Source: CAD feature listing. Evaluate the final solid. Frame: model axes, mm. Face numbers are marked on the shaded views. A direction names the side the tool comes from. Round coordinates to 2 decimals unless told otherwise and drop trailing zeros. Loops run counter-clockwise (first coordinate to the right, second up) from the corner with the lowest first, then second, coordinate; pieces in that order, holes last. Notation, with made-up numbers: (37.25, 29) -> (81.25, 29) arc R29 ccw to (81.25, 63) -> close; hole circle Ø1 at (-8.75, -8.75). An arc over 180 degrees is marked (long way). Write item = value, one per line.
from build123d import *
from OCP.BRepFilletAPI import BRepFilletAPI_MakeChamfer

# Parameters (mm, degrees)
SKETCH1_R                  = 2.2
SKETCH1_W                  = 22.4
SKETCH1_H                  = 25.8
BOSS_EXTRUDE1_DEPTH        = 42
CUT_EXTRUDE1_DEPTH         = 69.433909723
BOSS_EXTRUDE2_DEPTH        = 14.6
SKETCH4_W                  = 36
SKETCH4_H                  = 20
CUT_EXTRUDE2_DEPTH         = 18.2
SKETCH5_R                  = 2.2
CUT_EXTRUDE3_DEPTH         = 71.161242862
SKETCH16_W                 = 26.03
SKETCH16_H                 = 42
BOSS_EXTRUDE6_DEPTH        = 3
CHAMFER1_SIZE              = 7.42526056
CHAMFER1_SIZE_2            = 3
CHAMFER1_OF_MIRROR7_SIZE   = 7.42526056
CHAMFER1_OF_MIRROR7_SIZE_2 = 3
CUT_EXTRUDE4_START         = -1.9
CUT_EXTRUDE4_DEPTH         = 3.35
SKETCH10_R                 = 1.2
CUT_EXTRUDE10_DEPTH        = 72.637978754
SKETCH13_W                 = 22.4
SKETCH13_H                 = 1.9
BOSS_EXTRUDE4_DEPTH        = 1
SKETCH14_W                 = 3
SKETCH14_H                 = 7
CUT_EXTRUDE11_DEPTH        = 2.8
SKETCH15_W                 = 22.4
SKETCH15_H                 = 1.9
BOSS_EXTRUDE5_DEPTH        = 1
MIRROR5_START              = -1.9
MIRROR5_COPY_1_DEPTH       = 3.35
SKETCH17_W                 = 13.216816462
SKETCH17_H                 = 5
SKETCH17_W_2               = 8
BOSS_EXTRUDE7_DEPTH        = 3.2
FILLET1_SIZE               = 3
FILLET1_SIZE_2             = 18
FILLET3_SIZE               = 5
FILLET3_SIZE_2             = 4


# Some blends are built 0.0001 mm under size
with BuildPart() as part:
    # Sketch1 → Boss-Extrude1 (new body)
    with BuildSketch(Plane.XY):
        Polygon((2, 0), (45.2, 0), (45.2, 29.6), (2, 29.6), (0, 29.6), (0, 27.6), (0, 2), (0, 0), align=None)
        with Locations(Location((35.2, 14.8, 0), (0, 0, 180))):
            Circle(SKETCH1_R, mode=Mode.SUBTRACT)
        with Locations((13, 14.8)):
            Rectangle(SKETCH1_W, SKETCH1_H, mode=Mode.SUBTRACT)
    extrude(amount=BOSS_EXTRUDE1_DEPTH)

    # Sketch2 → Cut-Extrude1 (cut, through all)
    with BuildSketch(Plane(origin=(0, 29.6, 0), x_dir=(1, 0, 0), z_dir=(0, 1, 0))):
        Polygon((45.2, -26), (26.03, -42), (45.2, -42), align=None)
    extrude(amount=-CUT_EXTRUDE1_DEPTH, mode=Mode.SUBTRACT)

    # Sketch3 → Boss-Extrude2 (add)
    with BuildSketch(Plane(origin=(0, 0, 0), x_dir=(-1, 0, 0), z_dir=(0, 0, -1))):
        Polygon((-38.8, 0), (-45.2, -3.8), (-45.2, 0), align=None)
        Polygon((-45.2, 29.6), (-38.8, 29.6), (-45.2, 33.4), align=None)
    extrude(amount=-BOSS_EXTRUDE2_DEPTH)

    # Sketch4 → Cut-Extrude2 (cut)
    with BuildSketch(Plane(origin=(45.2, 0, 0), x_dir=(0, 0, -1), z_dir=(1, 0, 0))):
        with Locations((-24, 14.8)):
            Rectangle(SKETCH4_W, SKETCH4_H)
    extrude(amount=-CUT_EXTRUDE2_DEPTH, mode=Mode.SUBTRACT)

    # Sketch5 → Cut-Extrude3 (cut, through all)
    with BuildSketch(Plane(origin=(0, 29.6, 0), x_dir=(1, 0, 0), z_dir=(0, 1, 0))):
        with Locations(Location((35.2, -16, 0), (0, 0, 270))):
            Circle(SKETCH5_R)
    extrude(amount=-CUT_EXTRUDE3_DEPTH, mode=Mode.SUBTRACT)

    # Sketch16 → Boss-Extrude6 (add)
    with BuildSketch(Plane(origin=(0, 29.6, 0), x_dir=(1, 0, 0), z_dir=(0, 1, 0))):
        with Locations((13.015, -21)):
            Rectangle(SKETCH16_W, SKETCH16_H)
    boss_extrude6 = extrude(amount=BOSS_EXTRUDE6_DEPTH)

    # Chamfer1
    chamfer1_edges_1 = [part.edges().sort_by_distance(p)[0] for p in [
        (13.015, 32.6, 42),
    ]]
    chamfer1_side_1 = [part.faces().sort_by_distance(p)[0] for p in [
        (13.015, 32.6, 41.94),
    ]]
    chamfer1_edges_2 = [part.edges().sort_by_distance(p)[0] for p in [
        (26.03, 32.6, 21),
    ]]
    chamfer1_side_2 = [part.faces().sort_by_distance(p)[0] for p in [
        (26.03, 32.54, 21),
    ]]
    chamfer1_edges_3 = [part.edges().sort_by_distance(p)[0] for p in [
        (13.015, 32.6, 0),
    ]]
    chamfer1_side_3 = [part.faces().sort_by_distance(p)[0] for p in [
        (13.015, 32.6, 0.06),
    ]]
    chamfer1_edges_4 = [part.edges().sort_by_distance(p)[0] for p in [
        (0, 32.6, 21),
    ]]
    chamfer1_side_4 = [part.faces().sort_by_distance(p)[0] for p in [
        (0.06, 32.6, 21),
    ]]
    chamfer1 = BRepFilletAPI_MakeChamfer(part.part.solid().wrapped)
    for e in chamfer1_edges_1:
        chamfer1.Add(CHAMFER1_SIZE - 0.0001, CHAMFER1_SIZE_2 - 0.0001, e.wrapped, chamfer1_side_1[0].wrapped)
    for e in chamfer1_edges_2:
        chamfer1.Add(CHAMFER1_SIZE_2 - 0.0001, CHAMFER1_SIZE - 0.0001, e.wrapped, chamfer1_side_2[0].wrapped)
    for e in chamfer1_edges_3:
        chamfer1.Add(CHAMFER1_SIZE - 0.0001, CHAMFER1_SIZE_2 - 0.0001, e.wrapped, chamfer1_side_3[0].wrapped)
    for e in chamfer1_edges_4:
        chamfer1.Add(CHAMFER1_SIZE - 0.0001, CHAMFER1_SIZE_2 - 0.0001, e.wrapped, chamfer1_side_4[0].wrapped)
    add(Compound.cast(chamfer1.Shape()), mode=Mode.REPLACE)  # a hair under: the kernel refuses the full size

    # Mirror7: Boss-Extrude6 across plane
    add(boss_extrude6.mirror(Plane(origin=(0, 14.8, 0), x_dir=(0, 0, 1), z_dir=(0, -1, 0))))

    # Chamfer1 of Mirror7
    chamfer1_of_mirror7_edges_1 = [part.edges().sort_by_distance(p)[0] for p in [
        (13.015, -3, 42),
    ]]
    chamfer1_of_mirror7_side_1 = [part.faces().sort_by_distance(p)[0] for p in [
        (13.015, -3, 41.94),
    ]]
    chamfer1_of_mirror7_edges_2 = [part.edges().sort_by_distance(p)[0] for p in [
        (26.03, -3, 21),
    ]]
    chamfer1_of_mirror7_side_2 = [part.faces().sort_by_distance(p)[0] for p in [
        (26.03, -2.94, 21),
    ]]
    chamfer1_of_mirror7_edges_3 = [part.edges().sort_by_distance(p)[0] for p in [
        (13.015, -3, 0),
    ]]
    chamfer1_of_mirror7_side_3 = [part.faces().sort_by_distance(p)[0] for p in [
        (13.015, -2.94, 0),
    ]]
    chamfer1_of_mirror7_edges_4 = [part.edges().sort_by_distance(p)[0] for p in [
        (0, -3, 21),
    ]]
    chamfer1_of_mirror7_side_4 = [part.faces().sort_by_distance(p)[0] for p in [
        (0.06, -3, 21),
    ]]
    chamfer1_of_mirror7 = BRepFilletAPI_MakeChamfer(part.part.solid().wrapped)
    for e in chamfer1_of_mirror7_edges_1:
        chamfer1_of_mirror7.Add(CHAMFER1_OF_MIRROR7_SIZE - 0.0001, CHAMFER1_OF_MIRROR7_SIZE_2 - 0.0001, e.wrapped, chamfer1_of_mirror7_side_1[0].wrapped)
    for e in chamfer1_of_mirror7_edges_2:
        chamfer1_of_mirror7.Add(CHAMFER1_OF_MIRROR7_SIZE_2 - 0.0001, CHAMFER1_OF_MIRROR7_SIZE - 0.0001, e.wrapped, chamfer1_of_mirror7_side_2[0].wrapped)
    for e in chamfer1_of_mirror7_edges_3:
        chamfer1_of_mirror7.Add(CHAMFER1_OF_MIRROR7_SIZE_2 - 0.0001, CHAMFER1_OF_MIRROR7_SIZE - 0.0001, e.wrapped, chamfer1_of_mirror7_side_3[0].wrapped)
    for e in chamfer1_of_mirror7_edges_4:
        chamfer1_of_mirror7.Add(CHAMFER1_OF_MIRROR7_SIZE - 0.0001, CHAMFER1_OF_MIRROR7_SIZE_2 - 0.0001, e.wrapped, chamfer1_of_mirror7_side_4[0].wrapped)
    add(Compound.cast(chamfer1_of_mirror7.Shape()), mode=Mode.REPLACE)  # a hair under: the kernel refuses the full size

    # Sketch6 → Cut-Extrude4 (cut)
    with BuildSketch(Plane(origin=(0, 29.6, 0), x_dir=(1, 0, 0), z_dir=(0, 1, 0)).offset(CUT_EXTRUDE4_START)):
        Polygon((11.35, -13.4), (9.775198425, -10.5), (11.35, -7.6), (14.65, -7.6), (16.244163906, -10.5), (14.65, -13.4), align=None)
    cut_extrude4 = extrude(amount=CUT_EXTRUDE4_DEPTH, mode=Mode.SUBTRACT)

    # Sketch10 → Cut-Extrude10 (cut, through all)
    with BuildSketch(Plane(origin=(0, 32.6, 0), x_dir=(1, 0, 0), z_dir=(0, 1, 0))):
        with Locations(Location((13, -10.4, 0), (0, 0, 270))):
            Circle(SKETCH10_R)
    cut_extrude10 = extrude(amount=-CUT_EXTRUDE10_DEPTH, mode=Mode.SUBTRACT)

    # Mirror4: Cut-Extrude4 across plane
    add(cut_extrude4.mirror(Plane(origin=(0, 14.8, 0), x_dir=(0, 0, 1), z_dir=(0, -1, 0))), mode=Mode.SUBTRACT)

    # Sketch13 → Boss-Extrude4 (add)
    with BuildSketch(Plane.XY.offset(42)):
        with Locations((13, 2.85)):
            Rectangle(SKETCH13_W, SKETCH13_H)
        with Locations((13, 26.75)):
            Rectangle(SKETCH13_W, SKETCH13_H)
    extrude(amount=-BOSS_EXTRUDE4_DEPTH)

    # Sketch14 → Cut-Extrude11 (cut)
    with BuildSketch(Plane(origin=(27, 0, 0), x_dir=(0, 0, -1), z_dir=(1, 0, 0))):
        with Locations((-9.5, 14.8)):
            Rectangle(SKETCH14_W, SKETCH14_H)
        with Locations((-22.5, 14.8)):
            Rectangle(SKETCH14_W, SKETCH14_H)
    extrude(amount=-CUT_EXTRUDE11_DEPTH, mode=Mode.SUBTRACT)

    # Sketch15 → Boss-Extrude5 (add)
    with BuildSketch(Plane(origin=(0, 0, 0), x_dir=(-1, 0, 0), z_dir=(0, 0, -1))):
        with Locations((-13, 2.85)):
            Rectangle(SKETCH15_W, SKETCH15_H)
        with Locations((-13, 26.75)):
            Rectangle(SKETCH15_W, SKETCH15_H)
    extrude(amount=-BOSS_EXTRUDE5_DEPTH)

    # Mirror5: Cut-Extrude4, Cut-Extrude10 across plane
    add(cut_extrude4.mirror(Plane.XY.offset(21)), mode=Mode.SUBTRACT)
    add(cut_extrude10.mirror(Plane.XY.offset(21)), mode=Mode.SUBTRACT)

    # Mirror5 copy 1 sketch → Mirror5 copy 1 (cut)
    with BuildSketch(Plane(origin=(0, 0, 42), x_dir=(1, 0, 0), z_dir=(0, -1, 0)).offset(MIRROR5_START)):
        Polygon((11.35, -13.4), (9.775198425, -10.5), (11.35, -7.6), (14.65, -7.6), (16.244163906, -10.5), (14.65, -13.4), align=None)
    extrude(amount=MIRROR5_COPY_1_DEPTH, mode=Mode.SUBTRACT)

    # Sketch17 → Boss-Extrude7 (add)
    with BuildSketch(Plane.ZY.offset(-24.2)):
        with Locations((30.608408231, 14.8)):
            Rectangle(SKETCH17_W, SKETCH17_H)
        with Locations((4, 14.8)):
            Rectangle(SKETCH17_W_2, SKETCH17_H)
    extrude(amount=BOSS_EXTRUDE7_DEPTH)

    # Fillet1
    # a fillet whose section is not a circle: 18, 3 mm, written as the material it takes off along each edge
    with BuildSketch(Plane(origin=(21, 12.3, 24), x_dir=(1, 0, 0), z_dir=(0, 1, 0))) as fillet1_piece_1:
        with BuildLine():
            Bezier((FILLET1_SIZE, 0), (0, 0), (0, -FILLET1_SIZE_2), weights=[1, 0.538461538, 1])
            Line((0, -FILLET1_SIZE_2), (0, 0))
            Line((0, 0), (FILLET1_SIZE, 0))
        make_face()
    extrude(amount=5, mode=Mode.SUBTRACT)

    # Fillet2
    # a fillet whose section is not a circle: 1 mm, written as the material it takes off along each edge
    with BuildSketch(Plane(origin=(21.159285498, 19.997028117, 37.216816462), x_dir=(1, 0, 0), z_dir=(0, -1, 0))) as fillet2_piece_1:
        with BuildLine():
            Bezier((1.072400011, 0), (-0.006916058, 0), (0.075305906, -1.076179691), weights=[1, 1, 1])
            ThreePointArc((0.075305906, -1.076179691), (0.035933118, -0.538210194), (0, 0))
            Line((0, 0), (1.072400011, 0))
        make_face()
    extrude(amount=10.394056235, mode=Mode.SUBTRACT)

    # Fillet3
    # a fillet whose section is not a circle: 5, 4 mm, written as the material it takes off along each edge
    with BuildSketch(Plane(origin=(21, -0.2, 8), x_dir=(0, 0, -1), z_dir=(0, 1, 0))) as fillet3_piece_1_section:
        with BuildLine():
            Bezier((FILLET3_SIZE, 0), (0, 0), (0, -FILLET3_SIZE_2), weights=[1, 0.538461538, 1])
            Line((0, -FILLET3_SIZE_2), (0, 0))
            Line((0, 0), (FILLET3_SIZE, 0))
        make_face()
    fillet3_piece_1 = extrude(amount=30, mode=Mode.PRIVATE)
    fillet3_piece_1 = split(fillet3_piece_1, bisect_by=Plane(origin=(21, 18.3, 8), z_dir=(0, -1, 0)), keep=Keep.TOP, mode=Mode.PRIVATE)
    fillet3_piece_1 = split(fillet3_piece_1, bisect_by=Plane(origin=(21, 11.3, 8), z_dir=(0, 1, 0)), keep=Keep.TOP, mode=Mode.PRIVATE)
    add(fillet3_piece_1, mode=Mode.SUBTRACT)


solid = part.part
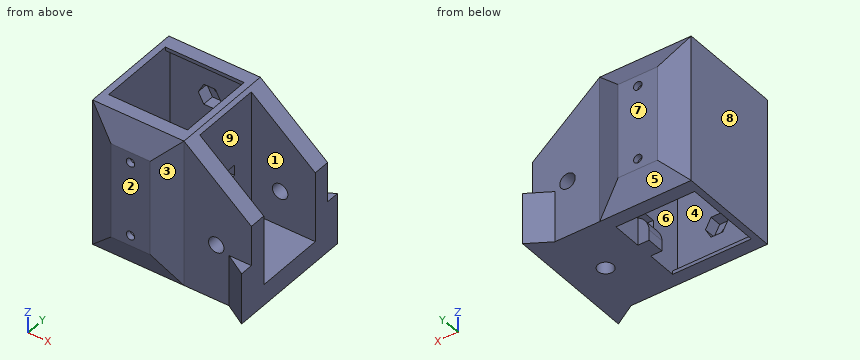
1. Section query A-A (z = 16). Give the number of separate pieces and of enclosed holes in the cut face, then the cut area to 3 significant figures.
Evaluation:
separate_pieces = 3
enclosed_holes = 1
area = 465 mm²
2. Section query B-B (x = 17.5). Return the cut outline in (y, z).
Evaluation:
outline = (-3, 7.43) -> (0, 0) -> (3.8, 0) -> (3.8, 1) -> (1.9, 1) -> (1.9, 41) -> (3.8, 41) -> (3.8, 42) -> (0, 42) -> (-3, 34.57) -> close; (25.8, 0) -> (29.6, 0) -> (32.6, 7.43) -> (32.6, 34.57) -> (29.6, 42) -> (25.8, 42) -> (25.8, 41) -> (27.7, 41) -> (27.7, 1) -> (25.8, 1) -> close
3. Section query D-D (x = 35.2). Return the cut outline in (y, z), then the cut area to 3 significant figures.
Evaluation:
outline = (0, 0) -> (12.6, 0) -> (12.6, 6) -> (4.8, 6) -> (4.8, 13.8) -> (0, 13.8) -> close; (0, 18.2) -> (4.8, 18.2) -> (4.8, 34.35) -> (0, 34.35) -> close; (17, 0) -> (29.6, 0) -> (29.6, 13.8) -> (24.8, 13.8) -> (24.8, 6) -> (17, 6) -> close; (24.8, 18.2) -> (29.6, 18.2) -> (29.6, 34.35) -> (24.8, 34.35) -> close
area = 381 mm²
4. Line query: probe 1 along X at (y, z) = (3, 16); probe 2 along Y at (x, z) = (10, 14); probe 3 along Y at (x, z) = (35.2, 2). Output: solid intervals per line, ascending. Write a range as from..to.
Evaluation:
probe_1 = 0..1.8, 24.2..33, 37.4..45.2
probe_2 = -3..1.9, 27.7..32.6
probe_3 = 0..12.6, 17..29.6
5. Section query C-C (y = 7.5). Return the cut outline in (x, z).
Evaluation:
outline = (0, 0) -> (1.8, 0) -> (1.8, 42) -> (0, 42) -> close; (24.2, 0) -> (45.2, 0) -> (45.2, 6) -> (27, 6) -> (27, 41.19) -> (26.03, 42) -> (24.2, 42) -> close
6. Contact query for flat-ended pins moving along their axis: pin 1 Ø9 at (x, z) = (11, 20) entering from -Y; pin 2 Ø18 at (x, z) = (18.5, 16) entering from +Y; pin 3 Ø15.5 at (x, z) = (36, 28) entering from -Y. Output: stop coordinate, or through.
Evaluation:
pin_1 = -3
pin_2 = 32.6
pin_3 = 0
7. Mould query, pull axis Y, two halves, no side actions, for the marked faces 6, 7, 8 and 9. Classes: released by +Y, released by -Y, zero draft, split by the parting line, or undercut.
Evaluation:
face_6 = undercut
face_7 = released by +Y
face_8 = zero draft
face_9 = undercut
8. Set-up query: the marked faces 1, 2, 3, 4 and 5. Return all of +Z, -Z, +X, -X, +Y, -Y with unobstructed straight access to the full face (end or side cutting, diameter ignored); none if empty.
Evaluation:
face_1 = +Z, +X
face_2 = +Z, -Z, -X, -Y
face_3 = +Z, -Z, -Y
face_4 = none
face_5 = -Z, -X, +Y
